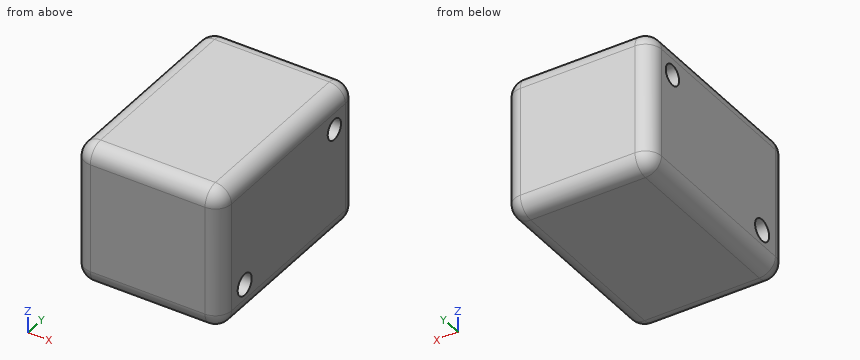
```python
from build123d import *

# Parameters (mm, degrees)
F0_W     = 45.763
F0_H     = 44.044
F1_DEPTH = 64.8
F2_R     = 5
F3_R     = 3.201525
F3_R_2   = 3.37016
F4_DEPTH = 124.6


with BuildPart() as f1:
    # F0 (on Front) → F1 (new body)
    with BuildSketch(Plane.XZ):
        Rectangle(F0_W, F0_H)
    extrude(amount=F1_DEPTH)

    # F2
    f2_edges = [f1.edges().sort_by_distance(p)[0] for p in [
        (22.8815, -32.4, 22.022),
        (-22.8815, -32.4, 22.022),
        (0, 0, 22.022),
        (0, -64.8, 22.022),
        (22.8815, -32.4, -22.022),
        (22.8815, 0, 0),
        (22.8815, -64.8, 0),
        (-22.8815, -32.4, -22.022),
        (-22.8815, 0, 0),
        (-22.8815, -64.8, 0),
        (0, 0, -22.022),
        (0, -64.8, -22.022),
    ]]
    fillet(f2_edges, radius=F2_R)

    # F3 (on face) → F4 (cut)
    with BuildSketch(Plane.YZ.offset(22.8815)):
        with Locations((-10.277459, 11.858958)):
            Circle(F3_R)
        with Locations((-53.430479, -12.360408)):
            Circle(F3_R_2)
    extrude(amount=-F4_DEPTH, mode=Mode.SUBTRACT)


solid = f1.part
```
Geometry check sheet. Reference: the model listing, model coordinates, mm. Give positions to 0.01 mm unless a question says otherwise; leave off trailing zeros. Loops run counter-clockwise (first coordinate to the right, second up) from the corner with the lowest first, then second, coordinate; pieces in that order, holes last. Notation, with made-up numbers: M 1,1 L 55,1 A27 ccw 55,39 Z; hole C 7.25,59 d5. An arc over 180 degrees is marked long. Write item = value, one per line.
(1) Sectioned sample at B-B, the plane x = -0.5. Record the cut outline in (y, z).
Answer below:
outline = M -64.8,-17.02 A5 ccw -59.8,-22.02 L -5,-22.02 A5 ccw 0,-17.02 L 0,17.02 A5 ccw -5,22.02 L -59.8,22.02 A5 ccw -64.8,17.02 Z; hole C -53.43,-12.36 d6.74; hole C -10.28,11.86 d6.4
(2) Sectioned sample at C-C, the plane y = -12.5. Record the cut outline in (x, z), plus the area to 3 significant figures.
Answer below:
outline = M -22.88,-17.02 A5 ccw -17.88,-22.02 L 17.88,-22.02 A5 ccw 22.88,-17.02 L 22.88,9.55 L -22.88,9.55 Z; M -22.88,14.16 L 22.88,14.16 L 22.88,17.02 A5 ccw 17.88,22.02 L -17.88,22.02 A5 ccw -22.88,17.02 Z
area = 1,780 mm2
(3) Sectioned sample at A-A, the plane z = -14. Record the cut outline in (x, y), plus the area to 3 significant figures.
Answer below:
outline = M -22.88,-59.8 A5 ccw -17.88,-64.8 L 17.88,-64.8 A5 ccw 22.88,-59.8 L 22.88,-56.37 L -22.88,-56.37 Z; M -22.88,-50.49 L 22.88,-50.49 L 22.88,-5 A5 ccw 17.88,0 L -17.88,0 A5 ccw -22.88,-5 Z
area = 2,670 mm2
(4) Sectioned sample at D-D, the plane z = 18.5. Record the cut outline in (x, y), plus the area to 3 significant figures.
Answer below:
outline = M -22.66,-59.8 A4.78 ccw -17.88,-64.58 L 17.88,-64.58 A4.78 ccw 22.66,-59.8 L 22.66,-5 A4.78 ccw 17.88,-0.22 L -17.88,-0.22 A4.78 ccw -22.66,-5 Z
area = 2,900 mm2
(5) Material ranges on line 1 (Z direction, x = 0.5, y = -53.5); line 2 (Z direction, x = -4, y = -12.5); line 3 (Y direction, x = 15, z = 9), recorded low to high. Write a range as [from, to].
Answer below:
line_1 = [-22.02, -15.73], [-8.99, 22.02]
line_2 = [-22.02, 9.55], [14.16, 22.02]
line_3 = [-64.8, -11.72], [-8.84, 0]
(6) Gauge pin test, flat ends, axial feed: pin 1 Ø5.5 at (y, z) = (-53.43, -12.36) entering from -X; pin 2 Ø10 at (y, z) = (-10.28, 11.86) entering from +X. Record the tip position at first contact, or that the pin passes through.
Answer below:
pin_1 = through
pin_2 = 22.88
